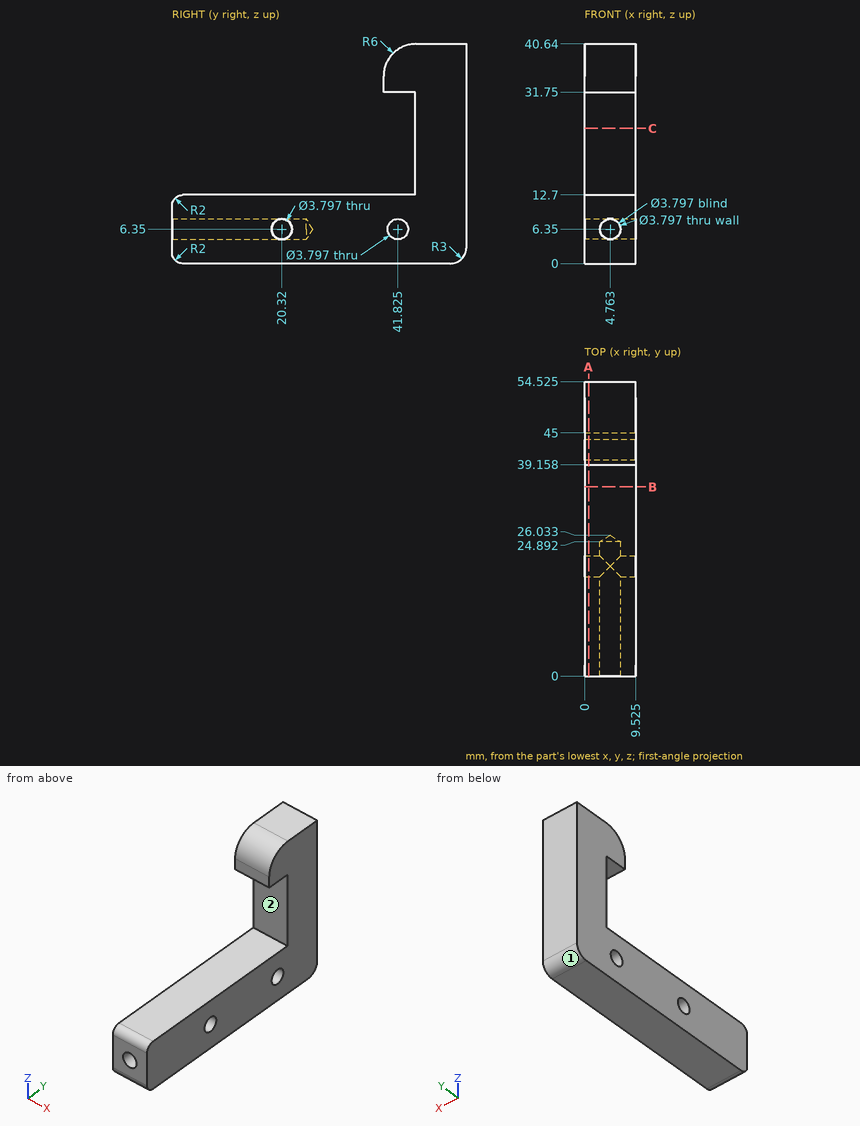
Source: three-view drawing plus pictorial views. Frame: mm from the lowest corner of the part. A direction names the side the tool comes from. Give positions to 0.01 mm unless a question says otherwise; leave off trailing zeros. Loops run counter-clockwise (first coordinate to the right, second up) from the corner with the lowest first, then second, coordinate; pieces in that order, holes last. Notation, with made-up numbers: (-0.5, 30) -> (20.5, 30) arc R23 cw to (20.5, 69) -> close; hole circle Ø5 at (-10.75, 22.25). An arc over 180 degrees is marked (long way). Put each result on its own line as item: value. Start each with the question number.
1) Cut plane B-B (y = 35). Return loops of the section in (x, z) (1 decimal).
2) Contact query for flat-ended pins moving along their axis: P1, Ø0.9, axis at x = 5, z = 33, coming from the -Y side; P2, Ø2.5, axis at y = 20.32, z = 6.35, coming from the +X side; P3, Ø2.5, axis at x = 4.76, z = 6.35, coming from the -Y side; P4, Ø3, axis at x = 6, z = 19.5, coming from the -Y side. Output: stop coordinate, or through.
3) Reachability of the marked faces 1 and 2 from +Z, -Z, +X, -X, +Y, -Y: full face, straight path, thin tool, end or side. Return the list, or none.
4) Cut plane A-A (x = 0.75). State how many separate pieces and enclosed holes the cut face has.
5) Material intervals for probe 1 along Z at (x, y) = (8, 20.32); probe 2 along Z at (x, y) = (5.5, 31.5); probe 3 along Y at (x, z) = (8.25, 21) (1 decimal), sorted ascending.
6) Cut plane C-C (z = 25). Return loops of the section in (x, y) (1 decimal).
Results are:
1. outline: (0, 0) -> (9.5, 0) -> (9.5, 12.7) -> (0, 12.7) -> close
2. P1: stops at y = 39.16
2. P2: passes through
2. P3: stops at y = 25.28
2. P4: stops at y = 45
3. face 1: -Z, +X, -X, +Y
3. face 2: +X, -X, -Y
4. separate pieces: 1
4. enclosed holes: 2
5. probe 1: z = 0 to 4.45, 8.25 to 12.7
5. probe 2: z = 0 to 12.7
5. probe 3: y = 45 to 54.5
6. outline: (0, 45) -> (9.5, 45) -> (9.5, 54.5) -> (0, 54.5) -> close
